Read the model definition and answer for the solid it produces. Units are mm, in the model's axes. Face numbers are marked on the shaded views. Round coordinates to 2 decimals unless told otherwise and drop trailing zeros. Order: outer loops, then holes, each group sorted by start corner. A loop starts at its lowest first (then second) coordinate and runs counter-clockwise, first axis right, second up. Notation, with made-up numbers: (3.5, 38) -> (62.5, 38) arc R20 cw to (62.5, 68) -> close; hole circle Ø6 at (57, 86.25). An arc over 180 degrees is marked (long way). Answer as a JSON object with one key per item and string values. Group by question number.
Item 1: Given P1, Ø3, axis at y = -7.5, z = 4, coming from the +X side; P2, Ø1.5, axis at y = 2.5, z = 1.5, coming from the -X side; P3, Ø1.5, axis at y = 5, z = 1.5, coming from the +X side, each flat-ended and moving along its own axis, determine where each tip first touches the part or whether it passes through.
Item 2: Consider probe 1 along Y at (x, z) = (0, 1.75) (3 decimals); probe 2 along Y at (x, z) = (-7, 2.4) (3 decimals); probe 3 along Y at (x, z) = (1, 0.8). Determine where each line is inside the solid, lowest interval first. Write a range as from..to.
Item 3: Section A-A, the plane y = 0 is taken. Write down the section's boundary in (x, z) (3 decimals).
Item 4: The mould has two halves that part along Y. Classify the marked faces 1, 2 and 3: pulls with the +Y half, pulls with the -Y half, needs draft (parallel to the pull), parting line crosses it, or undercut.
Item 5: Section C-C, the plane y = -7 is taken. Write down the section's boundary in (x, z) (3 decimals).
Item 6: Section D-D, the plane z = 3.85 is taken. Count the separate pieces of the cut face and the enclosed holes in it, plus the area to 3 significant figures.
Item 7: Section B-B, the plane x = -1.5 is taken. Write down the section's boundary in (y, z).
from build123d import *

# Parameters (mm, degrees)
ESQUISSE1_R        = 17.5
ESQUISSE1_R_2      = 0.925
ESQUISSE1_R_3      = 1.925
ESQUISSE1_R_4      = 4
BOSS_EXTRU_1_DEPTH = 5


with BuildPart() as part:
    # Esquisse1 → Boss.-Extru.1 (new body)
    with BuildSketch(Plane.XY):
        Circle(ESQUISSE1_R)
        with Locations((0, -7)):
            Circle(ESQUISSE1_R_2, mode=Mode.SUBTRACT)
        with Locations((-7, 0)):
            Circle(ESQUISSE1_R_2, mode=Mode.SUBTRACT)
        with Locations((0, 7)):
            Circle(ESQUISSE1_R_2, mode=Mode.SUBTRACT)
        with Locations((-7.25, -12.557368355)):
            Circle(ESQUISSE1_R_3, mode=Mode.SUBTRACT)
        with Locations((-7.25, 12.557368355)):
            Circle(ESQUISSE1_R_3, mode=Mode.SUBTRACT)
        Circle(ESQUISSE1_R_4, mode=Mode.SUBTRACT)
        with Locations((14.5, 0)):
            Circle(ESQUISSE1_R_3, mode=Mode.SUBTRACT)
        with Locations((7, 0)):
            Circle(ESQUISSE1_R_2, mode=Mode.SUBTRACT)
    extrude(amount=BOSS_EXTRU_1_DEPTH)


solid = part.part
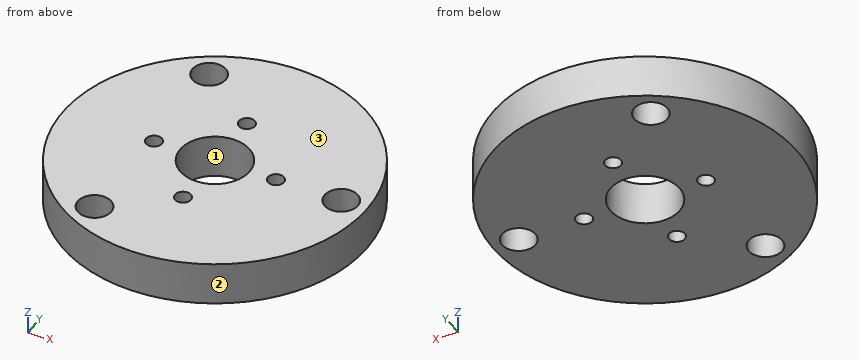
Values found:
{
 "1": {"P1": "x = 16.44", "P2": "x = -17.41", "P3": "x = 16.98"},
 "2": {"probe 1": "-17.5..-7.925, -6.075..-4, 4..6.075, 7.925..17.5", "probe 2": "-16.039..-14.466, -10.649..-0.925, 0.925..10.649, 14.466..16.039", "probe 3": "-17.47..-3.87, 3.87..17.47"},
 "3": {"outline": "(-17.5, 0) -> (-7.925, 0) -> (-7.925, 5) -> (-17.5, 5) -> close; (-6.075, 0) -> (-4, 0) -> (-4, 5) -> (-6.075, 5) -> close; (4, 0) -> (6.075, 0) -> (6.075, 5) -> (4, 5) -> close; (7.925, 0) -> (12.575, 0) -> (12.575, 5) -> (7.925, 5) -> close; (16.425, 0) -> (17.5, 0) -> (17.5, 5) -> (16.425, 5) -> close"},
 "4": {"face 1": "undercut", "face 2": "parting line crosses it", "face 3": "needs draft"},
 "5": {"outline": "(-16.039, 0) -> (-0.925, 0) -> (-0.925, 5) -> (-16.039, 5) -> close; (0.925, 0) -> (16.039, 0) -> (16.039, 5) -> (0.925, 5) -> close"},
 "6": {"separate pieces": "1", "enclosed holes": "8", "area": "866 mm2"},
 "7": {"outline": "(-17.44, 0) -> (-3.71, 0) -> (-3.71, 5) -> (-17.44, 5) -> close; (3.71, 0) -> (17.44, 0) -> (17.44, 5) -> (3.71, 5) -> close"}
}
